Print and shaded views of the part. All mm, measured from the part's lowest x, y and z. Coordinates: 2 decimals unless noted, no trailing zeros. Loops run counter-clockwise (first coordinate to the right, second up) from the corner with the lowest first, then second, coordinate; pieces in that order, holes last.
1) Wall check: line 1 along Y through (x, z) = (7, 5.5); line 2 along Z through (x, y) = (8.25, 3.75); line 3 along Y through (x, z) = (8.5, 40) (1 decimal). Give the ranges that are in metal, low to high.
2) Pin check, flat tips, straight feed: pin 1 Ø3 at (x, y) = (5.5, 5) entering from -Z; pin 2 Ø1 at (x, y) = (3, 3) entering from +Z; pin 3 Ø1.5 at (x, z) = (2.5, 31) entering from +Y. Stop position of each tip, or through.
3) Saw through at C-C, the plane z = 28. Write the cut outline in (x, y) (1 decimal).
4) Saw through at B-B, the plane y = 7. Write the cut outline in (x, z), and give its area (3 significant figures).
5) Two-plate mould, pull along Y, no slides. Class the marked faces 1, 2 and 3: +Y half, -Y half, draft (parallel to the pull), parting line (faces both ways), or undercut.
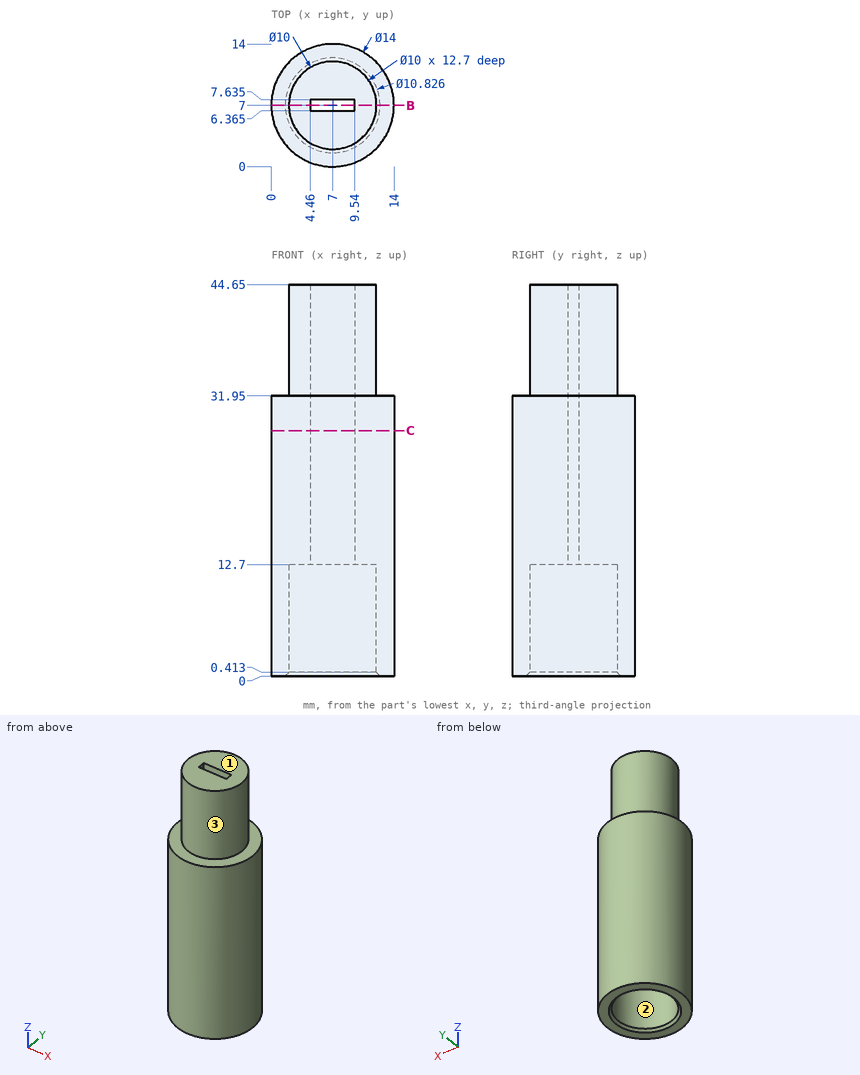
Data:
1. line 1: y = 0 to 2, 12 to 14
1. line 2: z = 12.7 to 44.65
1. line 3: y = 2.2 to 6.4, 7.6 to 11.8
2. pin 1: stops at z = 12.7
2. pin 2: stops at z = 31.95
2. pin 3: stops at y = 12.91
3. outline: circle Ø14 at (7, 7); hole (4.5, 6.4) - (9.5, 6.4) - (9.5, 7.6) - (4.5, 7.6) - close
4. outline: (0, 0) - (1.59, 0) - (2, 0.41) - (2, 12.7) - (4.46, 12.7) - (4.46, 44.65) - (2, 44.65) - (2, 31.95) - (0, 31.95) - close; (9.54, 12.7) - (12, 12.7) - (12, 0.41) - (12.41, 0) - (14, 0) - (14, 31.95) - (12, 31.95) - (12, 44.65) - (9.54, 44.65) - close
4. area: 285 mm2
5. face 1: draft
5. face 2: undercut
5. face 3: parting line
